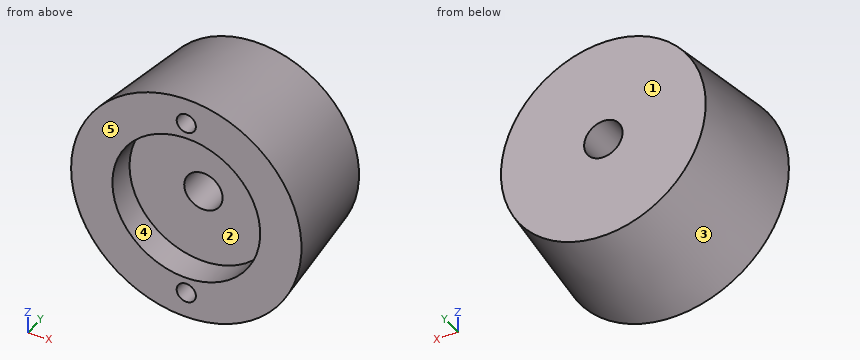
Autodesk Inventor part; units mm, degrees
ref_plane "YZ Plane" through (0, 0, 0) normal (1, 0, 0) x (0, 1, 0)
ref_plane "XZ Plane" through (0, 0, 0) normal (0, 1, 0) x (-1, 0, 0)
ref_plane "XY Plane" through (0, 0, 0) normal (0, 0, 1) x (1, 0, 0)
sketch "Esquisse1" plane through (0, 0, 0) normal (0, 0, 1) x (1, 0, 0)
  line L0 (-18, 0) -> (-16, 18.5)
  line L1 (-16, 18.5) -> (-3, 18.5)
  line L2 (-3, 18.5) -> (-3, 4.5)
  line L3 (-3, 4.5) -> (-11.55, 4.5)
  line L4 (-11.55, 4.5) -> (-11.55, 0)
  line L5 (-11.55, 0) -> (-18, 0)
  line L6 (0, -3.7) -> (0, 22.2) construction
  line L7 (-21.6, 0) -> (3.6, 0) construction
  point P0 (0, 0)
  dimension "d0" = 4.5
  dimension "d3" = 6
  dimension "d4" = 36
  dimension "d5" = 23.1
  dimension "d6" = 32
  dimension "d8" = 18.5
revolve "Révolution1" add sketch "Esquisse1" angle 360 about axis through (0, -10, 0) along (0, 1, 0)
sketch "Esquisse2" plane through (0, 0, 0) normal (0, -1, 0) x (1, 0, 0)
  circle A0 centre (0, 0) radius 14 construction
  circle A1 centre (0, -14) radius 1.5
  line L0 (0, -25.2) -> (0, 25.2) construction
  circle A2 centre (0, 14) radius 1.5
  dimension "d10" = 28
  dimension "d11" = 3
  dimension "d14" = 3
extrude "Extrusion1" cut sketch "Esquisse2" against normal blind 7
properties part number "bouton"
Work out the finished part from the listing and answer in its coordinate system (mm). Face numbers are marked on the shaded views. A direction names the side the tool comes from. Round coordinates to 2 decimals unless told otherwise and drop trailing zeros. Loops run counter-clockwise (first coordinate to the right, second up) from the corner with the lowest first, then second, coordinate; pieces in that order, holes last. Notation, with made-up numbers: (11, 78.25) - (45, 78.25) arc R27 ccw to (45, 113.25) - close; hole circle Ø5 at (23.25, 71). An arc over 180 degrees is marked (long way). One line per item, written item: value.
Q1. For the marked faces 4 and 5, determine the directions among +Z, -Z, +X, -X, +Y, -Y from which every point of the face is accessible in a straight line to the end or side of a thin tool.
Check values:
face 4: -Y
face 5: +Z, -Z, +X, -X, -Y
Q2. Find section C-C on y = 14.75. Give the vertices of the cut face in (x, z), and give its area (3 significant figures).
Check values:
outline: circle Ø32.81 at (0, 0); hole circle Ø6 at (0, 0)
area: 817 mm2
Q3. Find section D-D on y = 3.5. Give the vertices of the cut face in (x, z), and give its area (3 significant figures).
Check values:
outline: circle Ø35.24 at (0, 0); hole circle Ø23.1 at (0, 0); hole circle Ø3 at (0, -14); hole circle Ø3 at (0, 14)
area: 542 mm2
Q4. Each of these flat-tipped pins is pushed along its axis until it touches: pin 1 Ø8 at (x, y) = (-13.5, 6) entering from +Z; pin 2 Ø8 at (x, y) = (7, 15) entering from -Z; pin 3 Ø0.9 at (x, z) = (0, -14.5) entering from -Y. Where does it stop, or does it pass through?
Check values:
pin 1: z = 14.57
pin 2: z = -16.21
pin 3: y = 7
Q5. Find section A-A on z = 0. Give the vertices of the cut face in (x, y), and give its area (3 significant figures).
Check values:
outline: (-18, 0) - (-11.55, 0) - (-11.55, 4.5) - (-3, 4.5) - (-3, 18.5) - (-16, 18.5) - close; (3, 4.5) - (11.55, 4.5) - (11.55, 0) - (18, 0) - (16, 18.5) - (3, 18.5) - close
area: 441 mm2
Q6. Find section B-B on x = 0. Give the vertices of the cut face in (y, z).
Check values:
outline: (0, -18) - (18.5, -16) - (18.5, -3) - (4.5, -3) - (4.5, -11.55) - (0, -11.55) - (0, -12.5) - (7, -12.5) - (7, -15.5) - (0, -15.5) - close; (0, 11.55) - (4.5, 11.55) - (4.5, 3) - (18.5, 3) - (18.5, 16) - (0, 18) - (0, 15.5) - (7, 15.5) - (7, 12.5) - (0, 12.5) - close
Q7. The mould has two halves that part along Z. Classify the marked faces 1, 2 and 3: +Z half, -Z half, draft (parallel to the pull), parting line (faces both ways), or undercut.
Check values:
face 1: draft
face 2: undercut
face 3: parting line
Q8. Straight lines are drawn through the part: probe 1 along Z at (x, y) = (0, 1.7); probe 2 along X at (y, z) = (6.5, -13); probe 3 along Y at (x, z) = (-7.5, -8). For each, find the intervals that lie inside material, in ascending order.
Check values:
probe 1: -17.82 to -15.5, -12.5 to -11.55, 11.55 to 12.5, 15.5 to 17.82
probe 2: -11.41 to -1.12, 1.12 to 11.41
probe 3: 4.5 to 18.5
